Here's the drawing with two shaded views (mm, measured from the low corner). I have some questions. A direction names the side the tool comes from. Give positions to 0.01 mm unless a question says otherwise; leave off trailing zeros. Loops run counter-clockwise (first coordinate to the right, second up) from the corner with the lowest first, then second, coordinate; pieces in that order, holes last. Notation, with made-up numbers: M -32.75,57.25 L 18.25,57.25 A21 cw 18.25,70.25 Z; hole C 4,78 d4. An arc over 180 degrees is marked long. Use CSV: the item, a comma, the result in double quotes.
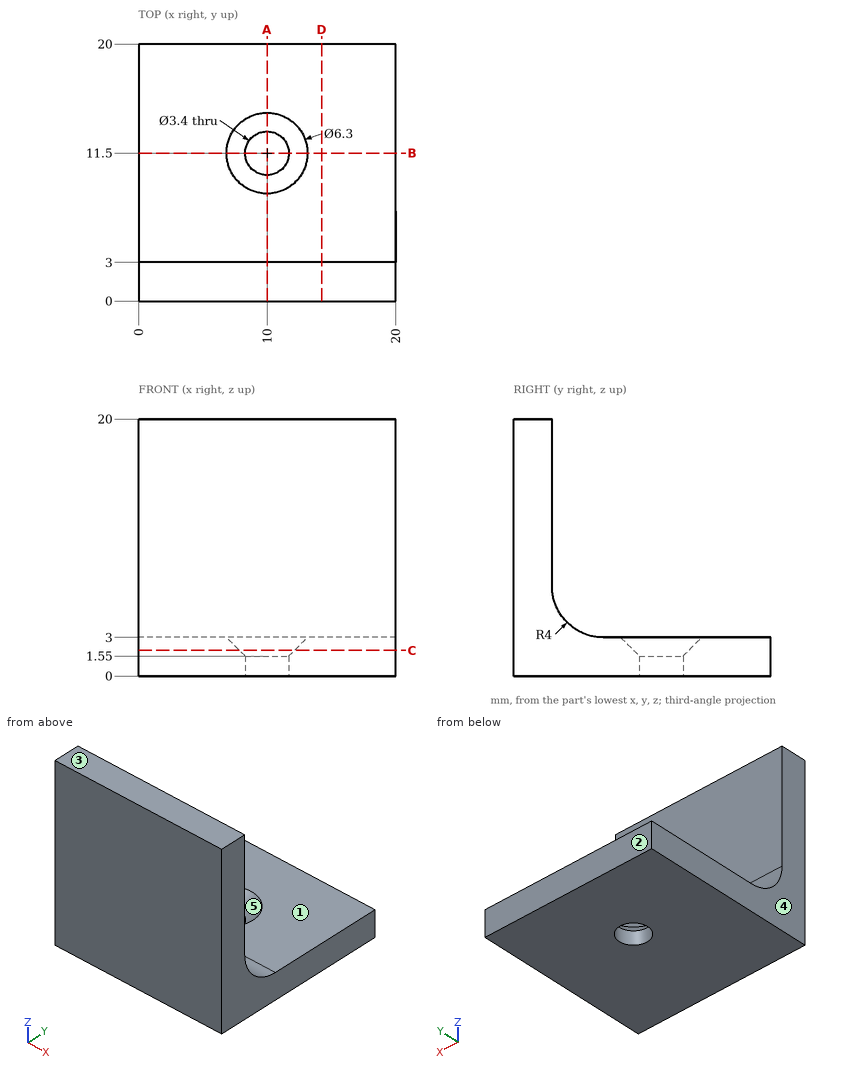
1. I want a section at D-D, the plane x = 14.25. List the corners of the cut face in (y, z) for me.
Outcome:
outline,"M 0,0 L 20,0 L 20,3 L 7,3 A4 cw 3,7 L 3,20 L 0,20 Z"
2. I'm going to push flat-ended pins straight in: pin 1 Ø10 at (x, z) = (8, 10) entering from +Y; pin 2 Ø5 at (x, y) = (7, 7) entering from +Z; pin 3 Ø4 at (x, y) = (3.5, 11) entering from +Z. Where does each tip first touch, or does it pass through?
Outcome:
pin 1,"y = 3.54"
pin 2,"z = 3.88"
pin 3,"z = 3"
3. I want a section at A-A, the plane x = 10. List the corners of the cut face in (y, z) for me, then the cut area to 3 significant figures.
Outcome:
outline,"M 0,0 L 9.8,0 L 9.8,1.55 L 8.35,3 L 7,3 A4 cw 3,7 L 3,20 L 0,20 Z; M 13.2,0 L 20,0 L 20,3 L 14.65,3 L 13.2,1.55 Z"
area,"102 mm2"
4. Which directions (+Z, -Z, +X, -X, +Y, -Y) give clear straight access to the entire face, cutting with the end or side of a thin tool? Please do the marked faces 1 and 2.
Outcome:
face 1,"+Z, +X, -X, +Y"
face 2,"+Z, -Z, +X, -X, +Y"
5. I want a section at B-B, the plane y = 11.5. List the corners of the cut face in (x, z) for me, then the cut area to 3 significant figures.
Outcome:
outline,"M 0,0 L 8.3,0 L 8.3,1.55 L 6.85,3 L 0,3 Z; M 11.7,0 L 20,0 L 20,3 L 13.15,3 L 11.7,1.55 Z"
area,"47.7 mm2"
6. I want a section at C-C, the plane z = 2. List the corners of the cut face in (x, y) for me.
Outcome:
outline,"M 0,0 L 20,0 L 20,20 L 0,20 Z; hole C 10,11.5 d4.3"
7. Please list where these lines run through material, in increasing order: line 1 (X direction, y = 11.5, z = 0.7); line 2 (Y direction, x = 10, z = 0.85); line 3 (Z direction, x = 4.75, y = 17.5).
Outcome:
line 1,"0 to 8.3, 11.7 to 20"
line 2,"0 to 9.8, 13.2 to 20"
line 3,"0 to 3"
8. If we mould it in two halves opening along X, with no side actions, what happens to the marked faces 3, 4 and 5? For each: +X half, -X half, draft (parallel to the pull), parting line (faces both ways), or undercut.
Outcome:
face 3,"draft"
face 4,"-X half"
face 5,"undercut"
